Print and shaded views of the part. All mm, measured from the part's lowest x, y and z. Coordinates: 2 decimals unless noted, no trailing zeros. Loops run counter-clockwise (first coordinate to the right, second up) from the corner with the lowest first, then second, coordinate; pieces in that order, holes last. Notation, with made-up numbers: M 45,-1 L 65,-1 A23 ccw 65,37 Z; hole C -7,13 d2. An arc over 180 degrees is marked long. Use a Markdown table: item, result. Add a question column.
1) Band-saw the part on A-A (y = 7.5). List the corners of the cut face in (x, z), plus the area to 3 significant figures.
2) Wall check: probe 1 along Y at (x, z) = (9, 2.05); probe 2 along X at (y, z) = (7.5, 1.7); probe 3 along X at (y, z) = (69.5, 1.85). Give the ranges that are in metal, low to high. Write a range as from..to.
3) Band-saw the part on B-B (x = 40.5). List the corners of the cut face in (y, z), plus the area to 3 significant figures.
4) Band-saw the part on C-C (y = 100). List the corners of the cut face in (x, z), plus the area to 3 significant figures.
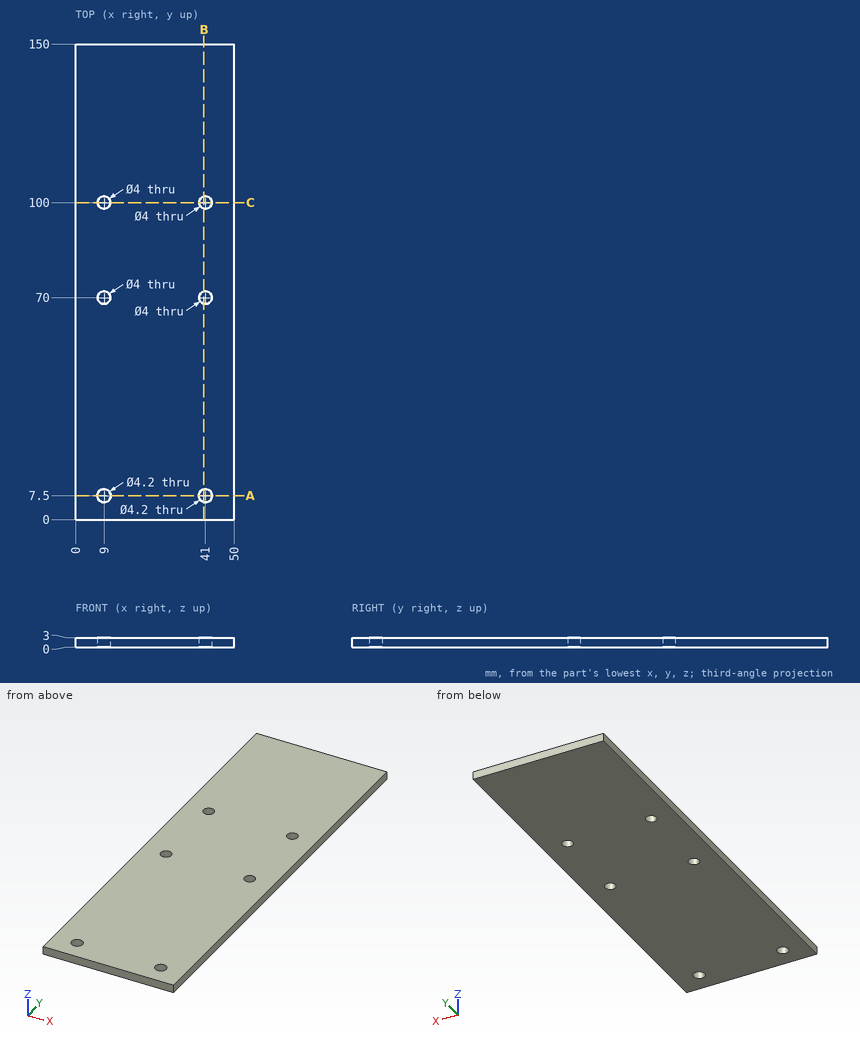
Entries:
| question | item | result |
|---|---|---|
| 1 | outline | M 0,0 L 6.9,0 L 6.9,3 L 0,3 Z; M 11.1,0 L 38.9,0 L 38.9,3 L 11.1,3 Z; M 43.1,0 L 50,0 L 50,3 L 43.1,3 Z |
| 1 | area | 125 mm2 |
| 2 | probe 1 | 0..5.4, 9.6..68, 72..98, 102..150 |
| 2 | probe 2 | 0..6.9, 11.1..38.9, 43.1..50 |
| 2 | probe 3 | 0..7.06, 10.94..39.06, 42.94..50 |
| 3 | outline | M 0,0 L 5.46,0 L 5.46,3 L 0,3 Z; M 9.54,0 L 68.06,0 L 68.06,3 L 9.54,3 Z; M 71.94,0 L 98.06,0 L 98.06,3 L 71.94,3 Z; M 101.94,0 L 150,0 L 150,3 L 101.94,3 Z |
| 3 | area | 415 mm2 |
| 4 | outline | M 0,0 L 7,0 L 7,3 L 0,3 Z; M 11,0 L 39,0 L 39,3 L 11,3 Z; M 43,0 L 50,0 L 50,3 L 43,3 Z |
| 4 | area | 126 mm2 |
